Design review of the part built by this model. Coordinates are the model's own, in mm. Face numbers are marked on the shaded views. A direction names the side the tool comes from. Give positions to 0.01 mm unless a question says otherwise; leave off trailing zeros. Write each loop counter-clockwise with the first axis right and the second up, starting at its lowest first coordinate (ties: lowest second). Pieces come first, ordered by that corner, then holes. Notation, with made-up numbers: (-3, -3) -> (49, -3) arc R22 cw to (49, 30) -> close; hole circle Ø4 at (45, 39). An arc over 180 degrees is marked (long way). Answer as a JSON object with one key per item and string values.
```python
from build123d import *

# Parameters (mm, degrees)
F0_W     = 65
F0_H     = 80.3
F1_DEPTH = 15.2
F2_R     = 5
F3_DEPTH = 120
F4_R     = 4.25
F5_DEPTH = 25
F6_W     = 20
F6_H     = 14.5
F6_R     = 3.75
F7_DEPTH = 10


with BuildPart() as f1:
    # F0 (on Top) → F1 (new body)
    with BuildSketch(Plane.XY):
        Rectangle(F0_W, F0_H)
    extrude(amount=F1_DEPTH)

    # F2 (on face) → F3 (join)
    with BuildSketch(Plane(origin=(0, 40.15, 0), x_dir=(-1, 0, 0), z_dir=(0, 1, 0))):
        with Locations((23, 6.9)):
            Circle(F2_R)
    extrude(amount=F3_DEPTH)

    # F4 (on face) → F5 (join)
    with BuildSketch(Plane.XZ.offset(40.15)):
        with Locations((-22.6, 7.6)):
            Circle(F4_R)
        with Locations((0, 7.6)):
            Circle(F4_R)
        with Locations((19.9, 9.3)):
            Circle(F4_R)
    extrude(amount=F5_DEPTH)

    # F6 (on face) → F7 (join)
    with BuildSketch(Plane.XY.offset(15.2)):
        with Locations((-12.5, -5.9)):
            Rectangle(F6_W, F6_H)
        with Locations((15.5, 1.35)):
            Circle(F6_R)
        with Locations((15.5, -13.65)):
            Circle(F6_R)
    extrude(amount=F7_DEPTH)


solid = f1.part
```
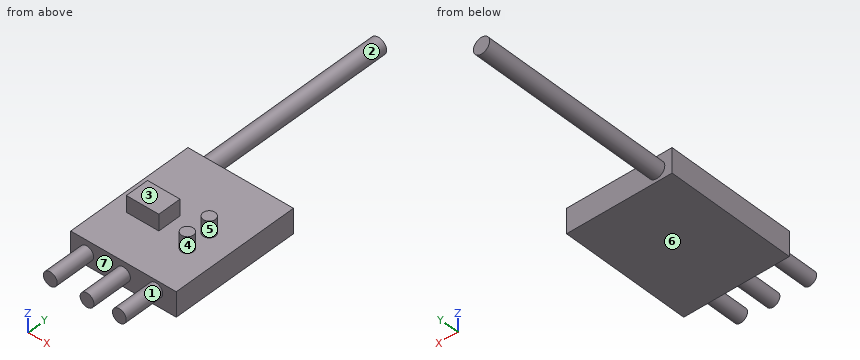
(1) The part is to be moulded in two halves that separate along Y. For the marked faces 4, 5, 6 and 7, say which applies: +Y half, -Y half, draft (parallel to the pull), parting line (faces both ways), or undercut.
Here are the results:
{"face 4": "undercut", "face 5": "undercut", "face 6": "draft", "face 7": "-Y half"}
(2) We need section B-B, the plane y = 55.5. State the section outline as (x, z) points, then the cut area to 3 significant figures.
Here are the results:
{"outline": "circle Ø10 at (-23, 6.9)", "area": "78.5 mm²"}
(3) We need section A-A, the plane x = 0. State the section outline as (y, z) points, then the cut area to 3 significant figures.
Here are the results:
{"outline": "(-65.15, 3.35) -> (-40.15, 3.35) -> (-40.15, 0) -> (40.15, 0) -> (40.15, 15.2) -> (-40.15, 15.2) -> (-40.15, 11.85) -> (-65.15, 11.85) -> close", "area": "1,430 mm²"}
(4) For line 1 along Y through (x, z) = (28, 4); line 2 along Z through (x, y) = (19.5, -3); line 3 along Y through (x, z) = (12.5, 18.25), list the stretches that pass through material, from the lowest coordinate up.
Here are the results:
{"line 1": "y = -40.15 to 40.15", "line 2": "z = 0 to 15.2", "line 3": "y = -15.9 to -11.4, -0.9 to 3.6"}
(5) We need section D-D, the plane y = -32.5. State the section outline as (x, z) points.
Here are the results:
{"outline": "(-32.5, 0) -> (32.5, 0) -> (32.5, 15.2) -> (-32.5, 15.2) -> close"}
(6) Clearance check with flat-ended pins moving along their axes: pin 1 (3 mm diameter, centred on x = 4, y = 30, fed in from +Z); pin 2 (5 mm diameter, centred on y = -8, z = 19, fed in from -X); pin 3 (3 mm diameter, centred on x = -16.5, z = 22.5, fed in from +Y). State where each tip first meets the part, or that it passes through.
Here are the results:
{"pin 1": "stops at z = 15.2", "pin 2": "stops at x = -22.5", "pin 3": "stops at y = 1.35"}
(7) For the marked faces 1, 2 and 3, list the 3-axis set-ups (+Z, -Z, +X, -X, +Y, -Y) from which the entire face can be reached by the end or side of a thin tool; tool diameter is ignored.
Here are the results:
{"face 1": "-Y", "face 2": "+Y", "face 3": "+Z, +X, -X, +Y, -Y"}
(8) We need section C-C, the plane x = -13. State the section outline as (y, z) points, then the cut area to 3 significant figures.
Here are the results:
{"outline": "(-40.15, 0) -> (40.15, 0) -> (40.15, 15.2) -> (1.35, 15.2) -> (1.35, 25.2) -> (-13.15, 25.2) -> (-13.15, 15.2) -> (-40.15, 15.2) -> close", "area": "1,370 mm²"}
